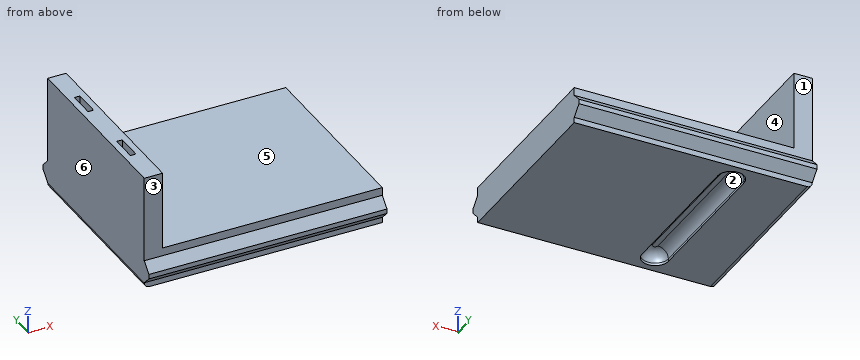
```python
from build123d import *

# Parameters (mm, degrees)
F0_W      = 90.6
F0_H      = 71.3
F1_DEPTH  = 14
F2_W      = 7
F2_H      = 71.3
F3_DEPTH  = 29.9
F5_DEPTH  = 90.6
F7_W      = 2.1
F7_H      = 10.1
F8_DEPTH  = 20.05
F9_R      = 5.04999
F10_R     = 2
F12_DEPTH = 5
F13_R     = 4


# Not quite as in the source:
# - a fillet or chamfer is up to 0.001 mm smaller than in the source, because OpenCascade refuses the exact size


with BuildPart() as f1:
    # F0 (on Top) → F1 (new body)
    with BuildSketch(Plane.XY):
        Rectangle(F0_W, F0_H)
    extrude(amount=F1_DEPTH)

    # F2 (on face) → F3 (join)
    with BuildSketch(Plane.XY.offset(14)):
        with Locations((-41.8, 0)):
            Rectangle(F2_W, F2_H)
    extrude(amount=F3_DEPTH)


with BuildPart() as f5:
    # F4 (on face) → F5 (new body)
    with BuildSketch(Plane.YZ.offset(45.3)):
        Polygon((-39.15, 5.6), (-35.65, 2.1), (-35.65, 10.9), (-39.15, 7.4), align=None)
    extrude(amount=-F5_DEPTH)


with BuildPart() as f5b:
    # F4 (on face) → F5, piece 2 (new body)
    with BuildSketch(Plane.YZ.offset(45.3)):
        Polygon((35.65, 10.9), (35.65, 2.1), (39.15, 5.6), (39.15, 7.4), align=None)
    extrude(amount=-F5_DEPTH)


with BuildPart() as f5_1:
    add(f5.part)

    # F6: union F1, F5b
    add(f1.part)
    add(f5b.part)

    # F7 (on face) → F8 (cut)
    with BuildSketch(Plane.XY.offset(43.9)):
        with Locations((-41.8, -15.65)):
            Rectangle(F7_W, F7_H)
        with Locations((-41.8, 15.65)):
            Rectangle(F7_W, F7_H)
    extrude(amount=-F8_DEPTH, mode=Mode.SUBTRACT)

    # F9 (radius 5.05 in the source; OpenCascade refuses exactly that, so slightly less here)
    f9_edges = [f5_1.edges().sort_by_distance(p)[0] for p in [
        (-41.8, -20.7, 23.85),
        (-41.8, -10.6, 23.85),
        (-41.8, 20.7, 23.85),
        (-41.8, 10.6, 23.85),
    ]]
    fillet(f9_edges, radius=F9_R)

    # F10
    f10_edges = [f5_1.edges().sort_by_distance(p)[0] for p in [
        (-45.3, 0, 0),
    ]]
    fillet(f10_edges, radius=F10_R)

    # F11 (on face) → F12 (cut)
    with BuildSketch(Plane(origin=(0, 0, 0), x_dir=(1, 0, 0), z_dir=(0, 0, -1))):
        with BuildLine():
            Line((-23.3, 28), (-23.3, -28))
            ThreePointArc((-23.3, -28), (-18.3, -33), (-13.3, -28))
            Line((-13.3, -28), (-13.3, 28))
            ThreePointArc((-13.3, 28), (-18.3, 33), (-23.3, 28))
        make_face()
    extrude(amount=-F12_DEPTH, mode=Mode.SUBTRACT)

    # F13
    f13_edges = [f5_1.edges().sort_by_distance(p)[0] for p in [
        (-23.3, 0, 5),
        (-18.3, 33, 5),
        (-13.3, 0, 5),
        (-18.3, -33, 5),
    ]]
    fillet(f13_edges, radius=F13_R)


solid = f5_1.part
```
Check sheet for the modelled part. Datum: model origin and axes. Units: mm. Face numbers are marked on the shaded views. A direction names the side the tool comes from. Give positions to 0.01 mm unless a question says otherwise; leave off trailing zeros. Write each loop counter-clockwise with the first axis right and the second up, starting at its lowest first coordinate (ties: lowest second). Pieces come first, ordered by that corner, then holes.
Item 1: Gauge pin test, flat ends, axial feed: pin 1 (0.6 mm diameter, centred on x = -42, z = 35.5, fed in from +Y); pin 2 (3 mm diameter, centred on y = 26, z = 28.5, fed in from +X); pin 3 (1 mm diameter, centred on x = -18.5, y = -12, fed in from -Z). Record the tip position at first contact, or that the pin passes through.
Item 2: Cross-section at A-A (y = 0). Enter the section's corners in (x, z).
Item 3: Draft check along Y on the marked faces 1, 2, 3 and 4. Enter one of: released by +Y, released by -Y, zero draft, split by the parting line, or undercut.
Item 4: Cross-section at B-B (x = 31.5). Enter the section's corners in (y, z).
Item 5: Cross-section at D-D (z = 9.5). Enter the section's corners in (x, y).
Item 6: Cross-section at C-C (z = 19). Enter the section's corners in (x, y), and give its area (3 significant figures).
Item 7: Scan lines: L1, parallel to Z at x = -13, y = -14; L2, parallel to X at y = -27, z = 20; L3, parallel to Y at x = -18, z = 11. Record each from-to range of solid material in increasing order.
Item 8: Access from +Z, -Z, +X, -X, +Y, -Y to the whole of each face (thin tool, end or side, straight path). Record for the marked faces 5 and 6.
Report:
1. pin 1: stops at y = 35.65
1. pin 2: stops at x = -38.3
1. pin 3: stops at z = 5
2. outline: (-45.3, 2) arc R2 ccw to (-43.3, 0) - (-23.3, 0) - (-23.3, 1) arc R4 cw to (-19.3, 5) - (-17.3, 5) arc R4 cw to (-13.3, 1) - (-13.3, 0) - (45.3, 0) - (45.3, 14) - (-38.3, 14) - (-38.3, 43.9) - (-45.3, 43.9) - close
3. face 1: released by +Y
3. face 2: undercut
3. face 3: released by -Y
3. face 4: zero draft
4. outline: (-39.15, 5.6) - (-35.65, 2.1) - (-35.65, 0) - (35.65, 0) - (35.65, 2.1) - (39.15, 5.6) - (39.15, 7.4) - (35.65, 10.9) - (35.65, 14) - (-35.65, 14) - (-35.65, 10.9) - (-39.15, 7.4) - close
5. outline: (-45.3, -37.05) - (45.3, -37.05) - (45.3, 37.05) - (-45.3, 37.05) - close
6. outline: (-45.3, -35.65) - (-38.3, -35.65) - (-38.3, 35.65) - (-45.3, 35.65) - close
6. area: 499 mm2
7. L1: z = 0 to 14
7. L2: x = -45.3 to -38.3
7. L3: y = -35.65 to 35.65
8. face 5: +Z, +X, +Y, -Y
8. face 6: +Z, -Z, -X, +Y, -Y
